```python
from build123d import *

# Parameters (mm, degrees)
F0_R          = 18.7710767317
F1_DEPTH      = 101.6
F2_R          = 21.1406607176
F3_DEPTH      = 14.986
F4_S5_R       = 18.7710767317
F4_T6_DEPTH   = 32
F5_SIZE2      = 1.27
F5_SIZE       = 1.27
F6_R          = 6.7296542148
F7_DEPTH      = 47.498
F7_DEPTH_BACK = 25.4


# Not quite as in the source:
# - a fillet or chamfer that OpenCascade refuses, or shapes differently, is made with other operations: its cross-section is extruded or revolved along the edge and cut away or added


with BuildPart() as f1:
    # F0 (on Front) → F1 (new body)
    with BuildSketch(Plane.XZ):
        Circle(F0_R)
    extrude(amount=-F1_DEPTH)

    # F2 (on Front) → F3 (join)
    with BuildSketch(Plane.XZ):
        Circle(F2_R)
    extrude(amount=F3_DEPTH)

    # F4: chamfer of 5.08 on 1 edges, made by hand


with BuildPart() as f4_tool2:
    # F4_s3 → F4_t4 (revolve)
    with BuildSketch(Plane.XY):
        Polygon((21.1406607176, -5.08), (16.0606607176, 0), (21.1406607176, 0), align=None)
    revolve(axis=Axis((0, 0, 0), (0, -1, 0)))

    # F4_s5 → F4_t6 (cut, symmetric)
    with BuildSketch(Plane.XZ.offset(2.5)):
        Circle(F4_S5_R)
    extrude(amount=F4_T6_DEPTH, both=True, mode=Mode.SUBTRACT)


with BuildPart() as f1_1:
    add(f1.part)

    # F4_t1: cut F4_tool2
    add(f4_tool2.part, mode=Mode.SUBTRACT)

    # F5
    f5_edges = [f1_1.edges().sort_by_distance(p)[0] for p in [
        (-21.140661, -14.986, 0),
    ]]
    chamfer(f5_edges, length=F5_SIZE, length2=F5_SIZE2)

    # F6 (on Right) → F7 (cut, two sides)
    with BuildSketch(Plane.YZ) as f7_sk:
        with Locations((76.0086998343, 0)):
            Circle(F6_R)
    extrude(amount=F7_DEPTH, mode=Mode.SUBTRACT)
    extrude(f7_sk.sketch, amount=-F7_DEPTH_BACK, mode=Mode.SUBTRACT)


solid = f1_1.part
```
Geometry check sheet. Reference: the model listing, model coordinates, mm. A direction names the side the tool comes from. Round coordinates to 2 decimals unless told otherwise and drop trailing zeros. Loops run counter-clockwise (first coordinate to the right, second up) from the corner with the lowest first, then second, coordinate; pieces in that order, holes last. Notation, with made-up numbers: M 61.25,64.25 L 87.25,64.25 A34 ccw 87.25,101.25 Z; hole C 0.25,-38.75 d6. An arc over 180 degrees is marked long. Return JSON: item names as keys, results as strings. Group by question number.
(1) Scan lines: line 1 along Y through (x, z) = (9.25, 0); line 2 along Y through (x, z) = (-14.5, 1); line 3 along Z through (x, y) = (-16, 72). Record each from-to range of solid material in increasing order. Write a range as [from, to].
(2) Section check B-B, the plane y = 61. Enter the section's corners in (x, z).
(3) Set-up check for faces 1 (the face through (0, -14.986, 0)), 2 (the face through (17.904, 48.715, 5.638)): record each of +Z, -Z, +X, -X, +Y, -Y from which the full face is reachable in a straight line by a thin tool's end or side.
(4) Go/stop test with flat-tipped pins: pin 1 (10 mm diameter, centred on y = 10.5, z = -12.5, fed in from -X); pin 2 (6 mm diameter, centred on y = 56.5, z = 12, fed in from -X); pin 3 (21.5 mm diameter, centred on y = 76.01, z = 0, fed in from +X). Record where each tip stops, or that it passes through.
(5) Section check A-A, the plane z = 0. Enter the section's corners in (x, y).
(6) Section check C-C, the plane y = 78. Enter the section's corners in (x, z), and give its area (3 significant figures).
Data:
{
 "1": {"line 1": "[-14.99, 69.28], [82.74, 101.6]", "line 2": "[-14.99, 69.35], [82.66, 101.6]", "line 3": "[-9.82, -5.41], [5.41, 9.82]"},
 "2": {"outline": "C 0,0 d37.54"},
 "3": {"face 1": "+Z, -Z, +X, -X, -Y", "face 2": "+Y"},
 "4": {"pin 1": "x = -17.21", "pin 2": "x = -16.47", "pin 3": "x = 18.77"},
 "5": {"outline": "M -21.14,-13.72 L -19.87,-14.99 L 19.87,-14.99 L 21.14,-13.72 L 21.14,-5.08 L 18.77,-2.71 L 18.77,69.28 L -18.77,69.28 L -18.77,-2.71 L -21.14,-5.08 Z; M -18.77,82.74 L 18.77,82.74 L 18.77,101.6 L -18.77,101.6 Z"},
 "6": {"outline": "M -17.64,-6.43 A18.77 ccw 17.64,-6.43 Z; M -17.64,6.43 L 17.64,6.43 A18.77 ccw Z", "area": "634 mm²"}
}
